Drawing for the job (mm, zero at the part's lowest x, y, z). A direction names the side the tool comes from. Give positions to 0.01 mm unless a question says otherwise; leave off trailing zeros. Order: outer loops, then holes, each group sorted by start corner. A loop starts at its lowest first (then second) coordinate and runs counter-clockwise, first axis right, second up. Notation, with made-up numbers: (-12.5, -23.75) - (2.5, -23.75) arc R16 cw to (2.5, -7.75) - close; hole circle Ø2 at (-34, -34). An arc over 180 degrees is marked (long way). One line per item, written item: value.
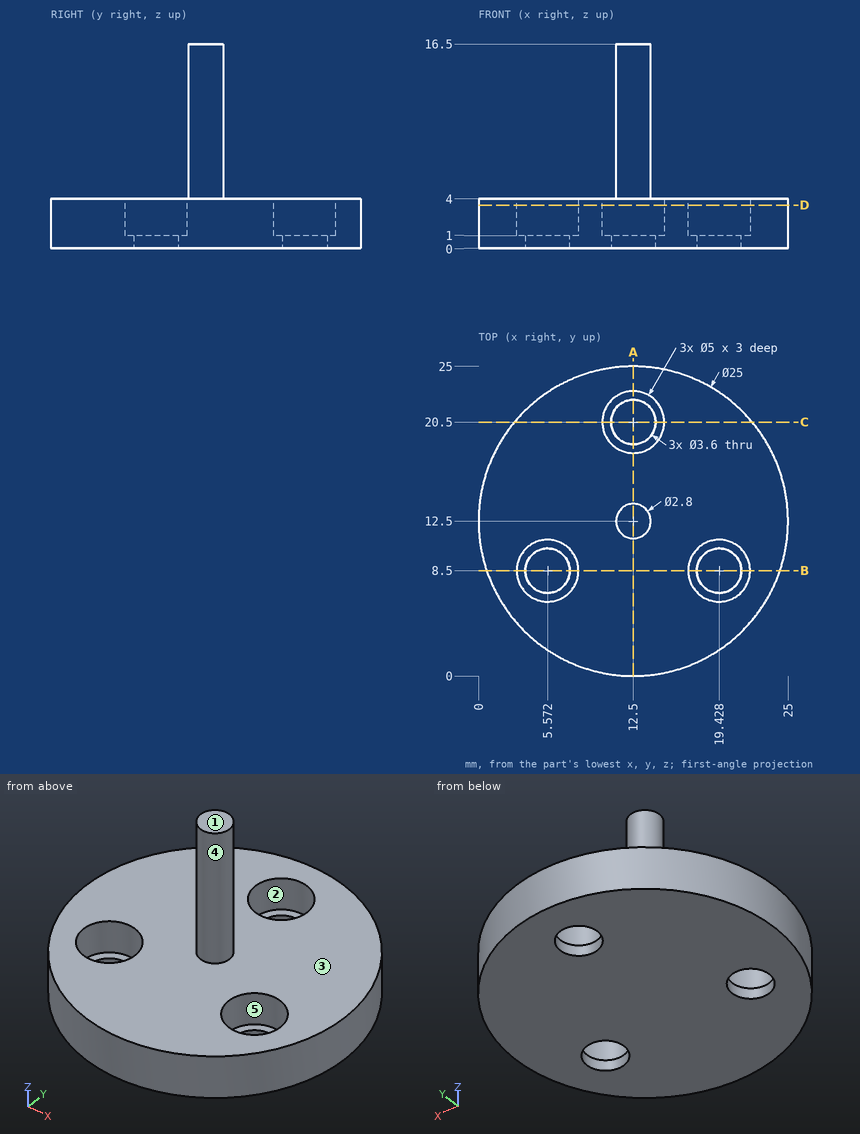
(1) Slice it at B-B, the plane y = 8.5. Give the cut face in (x, z).
Completed:
outline: (0.66, 0) - (3.77, 0) - (3.77, 1) - (3.07, 1) - (3.07, 4) - (0.66, 4) - close; (7.37, 0) - (17.63, 0) - (17.63, 1) - (16.93, 1) - (16.93, 4) - (8.07, 4) - (8.07, 1) - (7.37, 1) - close; (21.23, 0) - (24.34, 0) - (24.34, 4) - (21.93, 4) - (21.93, 1) - (21.23, 1) - close
(2) Drill centre lines: line 1 (Y direction, x = 12.5, z = 3.15); line 2 (Y direction, x = 12.5, z = 0.6); line 3 (X direction, y = 8.5, z = 0.35). Where is each one in solid material? Low to high.
Completed:
line 1: 0 to 18, 23 to 25
line 2: 0 to 18.7, 22.3 to 25
line 3: 0.66 to 3.77, 7.37 to 17.63, 21.23 to 24.34
(3) Slice it at A-A, the plane x = 12.5. Give the cut face in (y, z).
Completed:
outline: (0, 0) - (18.7, 0) - (18.7, 1) - (18, 1) - (18, 4) - (13.9, 4) - (13.9, 16.5) - (11.1, 16.5) - (11.1, 4) - (0, 4) - close; (22.3, 0) - (25, 0) - (25, 4) - (23, 4) - (23, 1) - (22.3, 1) - close
(4) Pull direction X, two halves, no side cores. Call the marked faces 3, 4 and 5: +X half, -X half, draft (parallel to the pull), parting line (faces both ways), or undercut.
Completed:
face 3: draft
face 4: parting line
face 5: undercut
(5) Slice it at C-C, the plane y = 20.5. Give the cut face in (x, z) (1 decimal).
Completed:
outline: (2.9, 0) - (10.7, 0) - (10.7, 1) - (10, 1) - (10, 4) - (2.9, 4) - close; (14.3, 0) - (22.1, 0) - (22.1, 4) - (15, 4) - (15, 1) - (14.3, 1) - close
(6) Slice it at D-D, the plane z = 3.5. Give the cut face in (x, y), and give its area (3 significant figures).
Completed:
outline: circle Ø25 at (12.5, 12.5); hole circle Ø5 at (5.57, 8.5); hole circle Ø5 at (12.5, 20.5); hole circle Ø5 at (19.43, 8.5)
area: 432 mm²
(7) 3-axis set-ups, long thin cutter, end or side, ignore diameter. For the marked faces 1 and 2: which of +Z, -Z, +X, -X, +Y, -Y reach the whole face in a straight line?
Completed:
face 1: +Z, +X, -X, +Y, -Y
face 2: +Z
(8) Pin check, flat tips, straight feed: P1, Ø3, axis at x = 12.5, y = 2.5, coming from the -Z side; P2, Ø2.5, axis at x = 19, y = 9, coming from the +Z side; P3, Ø5.5, axis at x = 12, y = 20, coming from the +Z side; P4, Ø2, axis at x = 6, z = 2, coming from the -Y side (1 decimal). Stop position of each tip, or through.
Completed:
P1: z = 0
P2: z = 1
P3: z = 4
P4: y = 1.3
